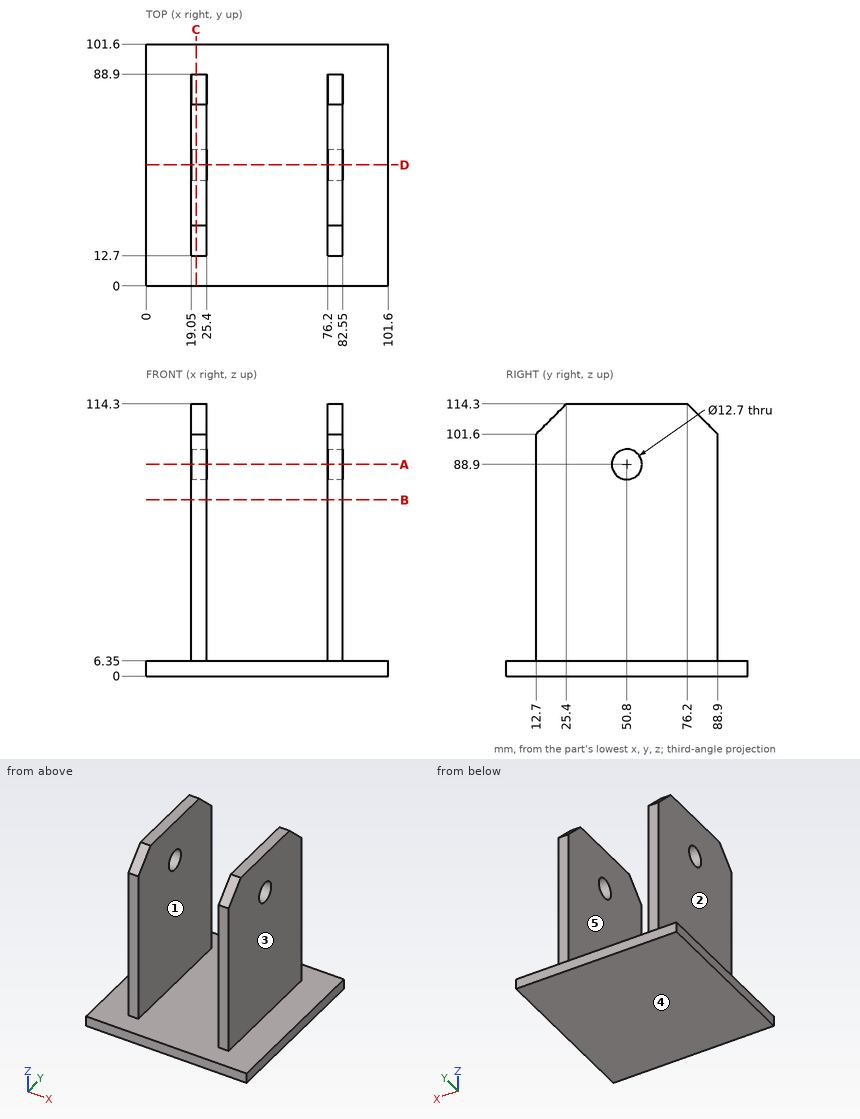
The figure shows three views and two pictorial views of one solid part (mm, origin at its lowest corner). Answer the questions. A direction names the side the tool comes from. Round coordinates to 2 decimals unless told otherwise and drop trailing zeros. Write each loop counter-clockwise with the first axis right and the second up, starting at its lowest first coordinate (ties: lowest second). Pieces come first, ordered by that corner, then holes. Notation, with made-up numbers: M -16.75,46.25 L 0.25,46.25 A25 cw 0.25,65.25 Z; hole C -14,42 d10. An arc over 180 degrees is marked long. Use a Markdown table: item, result.
1) The part is cut by section B-B (z = 74). Write down the section's boundary in (x, y).
Answers follow:
| item | result |
|---|---|
| outline | M 19.05,12.7 L 25.4,12.7 L 25.4,88.9 L 19.05,88.9 Z; M 76.2,12.7 L 82.55,12.7 L 82.55,88.9 L 76.2,88.9 Z |
2) A tool of negligible diameter and unlimited length cuts with its end or side. For the marked faces 4 and 5, from which of +Z, -Z, +X, -X, +Y, -Y can it reach the whole face along a straight path? Write none if from no direction.
Answers follow:
| item | result |
|---|---|
| face 4 | -Z, +X, -X, +Y, -Y |
| face 5 | +Z, +Y, -Y |
3) The part is cut by section A-A (z = 88.9). Write down the section's boundary in (x, y), plus the area to 3 significant figures.
Answers follow:
| item | result |
|---|---|
| outline | M 19.05,12.7 L 25.4,12.7 L 25.4,44.45 L 19.05,44.45 Z; M 19.05,57.15 L 25.4,57.15 L 25.4,88.9 L 19.05,88.9 Z; M 76.2,12.7 L 82.55,12.7 L 82.55,44.45 L 76.2,44.45 Z; M 76.2,57.15 L 82.55,57.15 L 82.55,88.9 L 76.2,88.9 Z |
| area | 806 mm2 |
4) Straight lines are drawn through the part: line 1 along Z through (x, y) = (79.5, 50.8); line 2 along X through (y, z) = (37, 13.5); line 3 along Z through (x, y) = (47.5, 61.5). For each, find the intervals that lie inside material, in ascending order. Write a range as [from, to].
Answers follow:
| item | result |
|---|---|
| line 1 | z = [0, 82.55], [95.25, 114.3] |
| line 2 | x = [19.05, 25.4], [76.2, 82.55] |
| line 3 | z = [0, 6.35] |
5) Flat-ended cylindrical pins translate along their axes: pin 1 (2 mm diameter, centred on y = 43, z = 47, fed in from +X); pin 2 (3 mm diameter, centred on x = 46, y = 72.5, fed in from +Z); pin 3 (5 mm diameter, centred on x = 78.5, z = 34.5, fed in from +Y); pin 4 (1.5 mm diameter, centred on x = 51.5, y = 39.5, fed in from -Z). Find the tip coordinate at first contact, or state that the pin passes through.
Answers follow:
| item | result |
|---|---|
| pin 1 | stops at x = 82.55 |
| pin 2 | stops at z = 6.35 |
| pin 3 | stops at y = 88.9 |
| pin 4 | stops at z = 0 |
6) The part is cut by section D-D (y = 50.8). Write down the section's boundary in (x, z).
Answers follow:
| item | result |
|---|---|
| outline | M 0,0 L 101.6,0 L 101.6,6.35 L 82.55,6.35 L 82.55,82.55 L 76.2,82.55 L 76.2,6.35 L 25.4,6.35 L 25.4,82.55 L 19.05,82.55 L 19.05,6.35 L 0,6.35 Z; M 19.05,95.25 L 25.4,95.25 L 25.4,114.3 L 19.05,114.3 Z; M 76.2,95.25 L 82.55,95.25 L 82.55,114.3 L 76.2,114.3 Z |
7) The part is cut by section C-C (x = 21). Write down the section's boundary in (y, z).
Answers follow:
| item | result |
|---|---|
| outline | M 0,0 L 101.6,0 L 101.6,6.35 L 88.9,6.35 L 88.9,101.6 L 76.2,114.3 L 25.4,114.3 L 12.7,101.6 L 12.7,6.35 L 0,6.35 Z; hole C 50.8,88.9 d12.7 |
8) For a pull along X with two mould halves and no side action, classify the marked faces 1, 2 and 3 as pulls with the +X half, pulls with the -X half, needs draft (parallel to the pull), parting line crosses it, or undercut.
Answers follow:
| item | result |
|---|---|
| face 1 | undercut |
| face 2 | pulls with the -X half |
| face 3 | pulls with the +X half |
